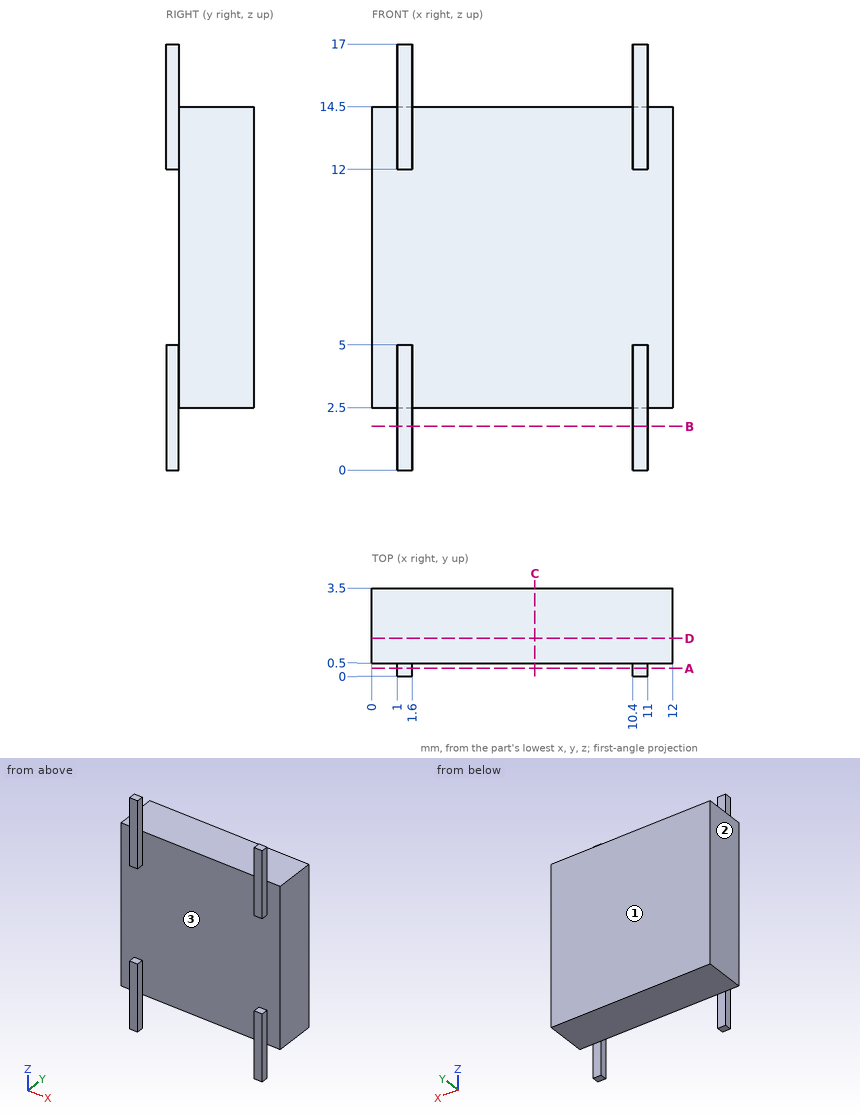
The drawing under review shows one solid part. Ordinate dimensions are in mm from its lowest x, y, z. Round coordinates to 2 decimals unless told otherwise and drop trailing zeros. Order: outer loops, then holes, each group sorted by start corner. A loop starts at its lowest first (then second) coordinate and runs counter-clockwise, first axis right, second up. Notation, with made-up numbers: (17, 62) -> (61, 62) arc R18 cw to (61, 97) -> close; hole circle Ø8 at (41, -35). An arc over 180 degrees is marked (long way). Use a Markdown table: item, result.
Item 1: Take a section at A-A (y = 0.3). State the section outline as (x, z) points.
Resolved:
| item | result |
|---|---|
| outline | (1, 0) -> (1.6, 0) -> (1.6, 5) -> (1, 5) -> close; (1, 12) -> (1.6, 12) -> (1.6, 17) -> (1, 17) -> close; (10.4, 0) -> (11, 0) -> (11, 5) -> (10.4, 5) -> close; (10.4, 12) -> (11, 12) -> (11, 17) -> (10.4, 17) -> close |
Item 2: For pin 1 (5 mm diameter, centred on x = 5, z = 11, fed in from -Y); pin 2 (0.7 mm diameter, centred on x = 1, z = 15.5, fed in from +Y); pin 3 (2 mm diameter, centred on x = 5, y = 1.5, fed in from +Z); pin 4 (0.6 mm diameter, centred on y = 0.5, z = 3, fed in from -X), all flat-tipped, find the tip position at first contact; note any pin that passes through.
Resolved:
| item | result |
|---|---|
| pin 1 | stops at y = 0.5 |
| pin 2 | stops at y = 0.5 |
| pin 3 | stops at z = 14.5 |
| pin 4 | stops at x = 0 |
Item 3: Take a section at C-C (x = 6.5). State the section outline as (y, z) points.
Resolved:
| item | result |
|---|---|
| outline | (0.5, 2.5) -> (3.5, 2.5) -> (3.5, 14.5) -> (0.5, 14.5) -> close |
Item 4: For line 1 along Z through (x, y) = (5.25, 1.8); line 2 along Y through (x, z) = (4.5, 10.5), list the stretches that pass through material, from the lowest coordinate up. Write a range as [from, to].
Resolved:
| item | result |
|---|---|
| line 1 | z = [2.5, 14.5] |
| line 2 | y = [0.5, 3.5] |
Item 5: Draft analysis for pull direction X (two halves, no side actions). For the marked faces 1, 2 and 3, state which applies: +X half, -X half, draft (parallel to the pull), parting line (faces both ways), or undercut.
Resolved:
| item | result |
|---|---|
| face 1 | draft |
| face 2 | -X half |
| face 3 | undercut |
Item 6: Take a section at D-D (y = 1.5). State the section outline as (x, z) points, plus the area to 3 significant figures.
Resolved:
| item | result |
|---|---|
| outline | (0, 2.5) -> (12, 2.5) -> (12, 14.5) -> (0, 14.5) -> close |
| area | 144 mm² |
Item 7: Take a section at B-B (z = 1.75). State the section outline as (x, y) points, plus the area to 3 significant figures.
Resolved:
| item | result |
|---|---|
| outline | (1, 0) -> (1.6, 0) -> (1.6, 0.5) -> (1, 0.5) -> close; (10.4, 0) -> (11, 0) -> (11, 0.5) -> (10.4, 0.5) -> close |
| area | 0.600 mm² |
